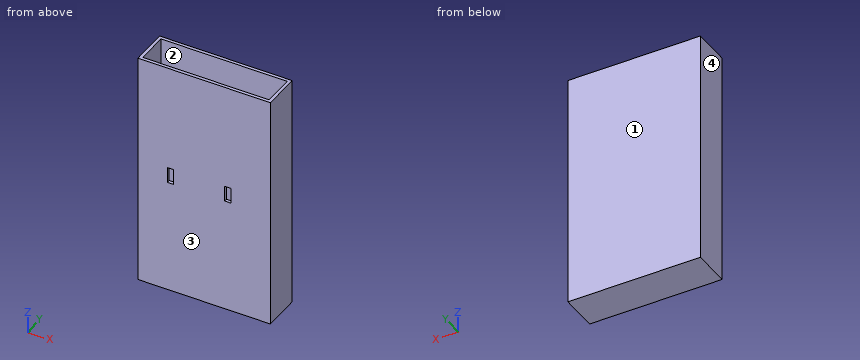
```python
from build123d import *

# Parameters (mm, degrees)
F1_W     = 84
F1_H     = 24
F2_DEPTH = 146
F3_DEPTH = 4
F0_W     = 80
F0_H     = 20
F4_DEPTH = 146
F5_W     = 4
F5_H     = 10
F6_DEPTH = 3.9


with BuildPart() as f2:
    # F1 (on Top) → F2 (new body)
    with BuildSketch(Plane.XY):
        Rectangle(F1_W, F1_H)
    extrude(amount=F2_DEPTH)

    # F1 (on Top) → F3 (join)
    with BuildSketch(Plane.XY):
        Rectangle(F1_W, F1_H)
    extrude(amount=-F3_DEPTH)

    # F0 (on Top) → F4 (cut)
    with BuildSketch(Plane.XY):
        Rectangle(F0_W, F0_H)
    extrude(amount=F4_DEPTH, mode=Mode.SUBTRACT)

    # F5 (on face) → F6 (cut)
    with BuildSketch(Plane.XZ.offset(12)):
        with Locations((-21.282188, 73.58651)):
            Rectangle(F5_W, F5_H)
        with Locations((15.067677, 73.934341)):
            Rectangle(F5_W, F5_H)
    extrude(amount=-F6_DEPTH, mode=Mode.SUBTRACT)


solid = f2.part
```
Part model, mm, in its own coordinate system. Face numbers are marked on the shaded views. Coordinates: 2 decimals unless noted, no trailing zeros. Write each loop counter-clockwise with the first axis right and the second up, starting at its lowest first coordinate (ties: lowest second). Pieces come first, ordered by that corner, then holes.
Item 1: Slice it at B-B (y = -1.25). Write the cut outline in (x, z), and give its area (3 significant figures).
Item 2: Mould opens along Y. For the marked faces 1, 2, 3 and 4 say: released by +Y, released by -Y, zero draft, split by the parting line, or undercut.
Item 3: Probe line 1 (X direction, y = 9.5, z = 45); line 2 (Y direction, x = 23, z = 6.5); line 3 (Z direction, x = 16.5, y = -11). List the from-to ranges inside material, lowest first.
Item 4: Slice it at C-C (x = 7). Write the cut outline in (y, z), and give its area (3 significant figures).
Item 5: Pin check, flat tip, straight feed: pin 1 (6 mm diameter, centred on x = -13.5, y = -0.5, fed in from +Z). Stop position of the tip, or through.
Item 6: Slice it at A-A (z = 51). Write the cut outline in (x, y).
Results found:
1. outline: (-42, -4) - (42, -4) - (42, 146) - (40, 146) - (40, 0) - (-40, 0) - (-40, 146) - (-42, 146) - close
1. area: 920 mm2
2. face 1: released by +Y
2. face 2: undercut
2. face 3: released by -Y
2. face 4: zero draft
3. line 1: x = -42 to -40, 40 to 42
3. line 2: y = -12 to -10, 10 to 12
3. line 3: z = -4 to 68.93, 78.93 to 146
4. outline: (-12, -4) - (12, -4) - (12, 146) - (10, 146) - (10, 0) - (-10, 0) - (-10, 146) - (-12, 146) - close
4. area: 680 mm2
5. pin 1: stops at z = 0
6. outline: (-42, -12) - (42, -12) - (42, 12) - (-42, 12) - close; hole (-40, -10) - (40, -10) - (40, 10) - (-40, 10) - close
